Could you check a few things on this model? Use its own coordinates, in mm. A direction names the side the tool comes from. Coordinates: 2 decimals unless noted, no trailing zeros. Order: outer loops, then holes, each group sorted by start corner. A loop starts at its lowest first (then second) coordinate and runs counter-clockwise, first axis right, second up. Notation, with made-up numbers: (41.5, 80.5) -> (45.5, 80.5) arc R28 cw to (45.5, 116.5) -> close; hole circle Ø4 at (43, 88). An arc over 180 degrees is marked (long way). Put each result on its own line as item: value. Start each with the question number.
Q1. If we section it at B-B (y = -16.5): Please give me the cut outline in (x, z), and give its area (3 significant figures).
Q2. Will these pins go through, and if not, where does the flat tip stop? pin 1 (5 mm diameter, centred on x = -3, z = -11.5, fed in from -Y); pin 2 (1.5 mm diameter, centred on x = 4.5, z = -23.5, fed in from +Y); pin 3 (2 mm diameter, centred on x = 1, y = 1.5, fed in from -Z).
Q3. Please list where these lines run through material, in increasing order: line 1 along Y through (x, z) = (-1, -10.25); line 2 along Z through (x, y) = (-2, -14); line 3 along X through (y, z) = (23.5, 1.25).
Q4. If we section it at D-D (x = 5): Please give me the cut outline in (y, z).
Q5. For faces 4 (the face through (0, 27, -14)), 5 (the face through (5, 28.5, -25.7)), 6 (the face through (-1.7, 0, 1)), which set-ups out of +Z, -Z, +X, -X, +Y, -Y let a thin tool reach every point of the face, with its end or its side?
Q6. If we section it at C-C (z = -19): Please give me the cut outline in (x, y).
Q7. If we section it at A-A (x = 0): Please give me the cut outline in (y, z), and give its area (3 significant figures).
Q8. We'd pull the mould along X, two halves only. Please class faces 1 (the face through (6.7, 29, -18)), 2 (the face through (0, -30, 1)), 3 (the face through (-10, 6.8, 0.3)): +X half, -X half, draft (parallel to the pull), parting line (faces both ways), or undercut.
Autodesk Inventor part; units mm, degrees
ref_plane "YZ Plane" through (0, 0, 0) normal (1, 0, 0) x (0, 1, 0)
ref_plane "XZ Plane" through (0, 0, 0) normal (0, 1, 0) x (-1, 0, 0)
ref_plane "XY Plane" through (0, 0, 0) normal (0, 0, 1) x (1, 0, 0)
sketch "Skizze1" plane through (0, 0, 0) normal (0, 0, 1) x (1, 0, 0)
  line L0 (-10, 30) -> (10, 30)
  line L1 (10, 30) -> (10, -30)
  line L2 (10, -30) -> (-10, -30)
  line L3 (-10, -30) -> (-10, 30)
  line L4 (-14, 0) -> (14, 0)
  line L5 (0, -42) -> (0, 42)
  line L6 (1.7, 24) -> (1.7, -24)
  line L7 (-1.7, -24) -> (-1.7, 24)
  arc A0 (1.7, 24) -> (-1.7, 24) centre (0, 24) ccw
  arc A1 (-1.7, -24) -> (1.7, -24) centre (0, -24) ccw
  point P0 (0, 0)
  dimension "d0" = 20
  dimension "d1" = 3.4
  dimension "d2" = 60
  dimension "d3" = 48
extrude "Extrusion1" add sketch "Skizze1" along normal blind 3 contours L0 L5 A0 L7 L4 L3 | L0 L1 L4 L6 A0 L5 | L4 L7 A1 L5 L2 L3 | L1 L2 L5 A1 L6 L4
sketch "Skizze2" plane through (10, -30, 0) normal (1, 0, 0) x (0, 0, -1)
  line L0 (-3, 60) -> (-3, 0)
  line L1 (0, 60) -> (27, 60)
  line L2 (27, 60) -> (27, 57)
  line L3 (27, 57) -> (0, 57)
  line L4 (0, 57) -> (0, 60)
  point P0 (0, 30)
  dimension "d6" = 3
  dimension "d7" = 30
extrude "Extrusion2" add sketch "Skizze2" against normal up to surface (20 mm away)
sketch "Skizze3" plane through (-10, 30, 3) normal (0, 1, 0) x (1, 0, 0)
  line L0 (0, 0) -> (20, 0)
  line L1 (20, 30) -> (0, 30)
  line L2 (10, 30) -> (10, 0)
  line L3 (13, 30) -> (17, 30)
  line L4 (17, 30) -> (17, 18.0571)
  line L5 (17, 18.0571) -> (13, 18.0571)
  line L6 (13, 18.0571) -> (13, 30)
  line L7 (16.7, 27) -> (16.7, 15)
  line L8 (13.3, 15) -> (13.3, 27)
  arc A0 (16.7, 27) -> (13.3, 27) centre (15, 27) ccw
  arc A1 (13.3, 15) -> (16.7, 15) centre (15, 15) ccw
  line L9 (15, 27) -> (15, 15)
  point P0 (10, 3)
  dimension "d10" = 3
  dimension "d11" = 4
  dimension "d12" = 2
  dimension "d13" = 3.4
  dimension "d14" = 3
  dimension "d15" = 12
extrude "Extrusion3" cut sketch "Skizze3" against normal blind 3 contours L7 A1 L8 L5 | L5 L8 A0 L7
properties part number "13_0204_065"
The answers:
1. outline: (-10, 0) -> (-1.7, 0) -> (-1.7, 3) -> (-10, 3) -> close; (1.7, 0) -> (10, 0) -> (10, 3) -> (1.7, 3) -> close
1. area: 49.8 mm^2
2. pin 1: y = 27
2. pin 2: through
2. pin 3: z = 0
3. line 1: 27 to 30
3. line 2: 0 to 3
3. line 3: -10 to -1.7, 1.7 to 10
4. outline: (-30, 0) -> (27, 0) -> (27, -10.3) -> (30, -10.3) -> (30, 3) -> (-30, 3) -> close; (27, -27) -> (30, -27) -> (30, -25.7) -> (27, -25.7) -> close
5. face 4: -Z, +X, -X, -Y
5. face 5: +Y, -Y
5. face 6: +Z, -Z
6. outline: (-10, 27) -> (3.3, 27) -> (3.3, 30) -> (-10, 30) -> close; (6.7, 27) -> (10, 27) -> (10, 30) -> (6.7, 30) -> close
7. outline: (-30, 0) -> (-25.7, 0) -> (-25.7, 3) -> (-30, 3) -> close; (25.7, 0) -> (27, 0) -> (27, -27) -> (30, -27) -> (30, 3) -> (25.7, 3) -> close
7. area: 107 mm^2
8. face 1: undercut
8. face 2: draft
8. face 3: -X half
